from build123d import *
from build123d.topology import SkipClean

# Parameters (mm, degrees)
BOSS_EXTRUDE1_DEPTH     = 1.5875
FILLET1_R               = 6.35
BOSS_EXTRUDE2_DEPTH     = 1.5875
FILLET2_R               = 3.175
CUT_EXTRUDE1_DEPTH      = 107.31034378
CUT_EXTRUDE1_DEPTH_BACK = 107.31034378
SKETCH3_R               = 1.5875


with BuildPart() as part:
    # Sketch1 → Boss-Extrude1 (new, symmetric)
    with SkipClean():  # the faces are left unmerged after this step: merging them gives an invalid solid
        with BuildSketch(Plane(origin=(0, 0, 0), x_dir=(0, 0, -1), z_dir=(1, 0, 0))):
            with BuildLine():
                Line((-38.1, -3.698033758), (-9.463093909, -3.698033758))
                ThreePointArc((-9.463093909, -3.698033758), (-10.16, 0), (-9.463093909, 3.698033758))
                Line((-9.463093909, 3.698033758), (-38.1, 3.698033758))
                ThreePointArc((-38.1, 3.698033758), (-41.798033758, 0), (-38.1, -3.698033758))
            make_face()
            with BuildLine():
                Line((-9.463093909, -3.698033758), (0, -3.698033758))
                ThreePointArc((0, -3.698033758), (-3.698033758, 0), (0, 3.698033758))
                Line((0, 3.698033758), (-9.463093909, 3.698033758))
                ThreePointArc((-9.463093909, 3.698033758), (-10.16, 0), (-9.463093909, -3.698033758))
            make_face()
            with BuildLine():
                Line((-9.463093909, 3.698033758), (0, 3.698033758))
                Line((0, 3.698033758), (9.463093909, 3.698033758))
                ThreePointArc((9.463093909, 3.698033758), (0, 10.16), (-9.463093909, 3.698033758))
            make_face()
            with BuildLine():
                Line((9.463093909, -3.698033758), (0, -3.698033758))
                Line((0, -3.698033758), (-9.463093909, -3.698033758))
                ThreePointArc((-9.463093909, -3.698033758), (0, -10.16), (9.463093909, -3.698033758))
            make_face()
            with BuildLine():
                ThreePointArc((0, 3.698033758), (3.698033758, 0), (0, -3.698033758))
                Line((0, -3.698033758), (9.463093909, -3.698033758))
                ThreePointArc((9.463093909, -3.698033758), (9.984253455, -1.881563962), (10.16, 0))
                ThreePointArc((10.16, 0), (9.984253455, 1.881563962), (9.463093909, 3.698033758))
                Line((9.463093909, 3.698033758), (0, 3.698033758))
            make_face()
            with BuildLine():
                ThreePointArc((10.16, 0), (9.984253455, -1.881563962), (9.463093909, -3.698033758))
                Line((9.463093909, -3.698033758), (101.6, -3.698033758))
                ThreePointArc((101.6, -3.698033758), (105.298033758, 0), (101.6, 3.698033758))
                Line((101.6, 3.698033758), (9.463093909, 3.698033758))
                ThreePointArc((9.463093909, 3.698033758), (9.984253455, 1.881563962), (10.16, 0))
            make_face()
        extrude(amount=BOSS_EXTRUDE1_DEPTH, both=True)

    # Fillet1
    fillet1_edges = [part.edges().sort_by_distance(p)[0] for p in [
        (0, -3.698033758, 9.463093909),
        (0, 3.698033758, 9.463093909),
        (0.79375, 3.698033758, -9.463093909),
        (0.79375, -3.698033758, -9.463093909),
    ]]
    fillet(fillet1_edges, radius=FILLET1_R)

    # Sketch2 → Boss-Extrude2 (add, symmetric)
    with SkipClean():  # the faces are left unmerged after this step: merging them gives an invalid solid
        with BuildSketch(Plane(origin=(0, 0, 0), x_dir=(0, 0, -1), z_dir=(1, 0, 0))):
            with BuildLine():
                Line((105.298033758, 0), (105.298033758, 12.7))
                ThreePointArc((105.298033758, 12.7), (103.756361287, 14.286838394), (102.125679632, 12.79161686))
                Line((102.125679632, 12.79161686), (101.6, 3.698033758))
                ThreePointArc((101.6, 3.698033758), (104.214904747, 2.614904747), (105.298033758, 0))
            make_face()
        extrude(amount=BOSS_EXTRUDE2_DEPTH, both=True)

    # Fillet2
    # the kernel refuses this fillet: 3.175 mm, written as the material it adds along each edge
    with BuildSketch(Plane(origin=(1.5875, 3.698033758, -101.6), x_dir=(0, 0, 1), z_dir=(-1, 0, 0))) as fillet2_piece_1:
        with BuildLine():
            CenterArc((FILLET2_R * 0.943861718873, FILLET2_R), FILLET2_R, 183.308458381, 86.691541619)
            Line((-FILLET2_R * 0.0544715888813, FILLET2_R * 0.942288591865), (0, 0))
            Line((0, 0), (FILLET2_R * 0.943861718873, 0))
        make_face()
    extrude(amount=3.175)

    # Sketch3 → Cut-Extrude1 (cut, two sides: drawn at the far end of the back side and taken through both)
    with BuildSketch(Plane(origin=(1.5875, 0, 0), x_dir=(0, 0, -1), z_dir=(1, 0, 0)).offset(-CUT_EXTRUDE1_DEPTH_BACK)):
        with Locations((-38.1, 0)):
            Circle(SKETCH3_R)
    extrude(amount=CUT_EXTRUDE1_DEPTH + CUT_EXTRUDE1_DEPTH_BACK, mode=Mode.SUBTRACT)


solid = part.part
Check sheet for the modelled part. Datum: model origin and axes. Units: mm. A direction names the side the tool comes from. Coordinates: 2 decimals unless noted, no trailing zeros. Write each loop counter-clockwise with the first axis right and the second up, starting at its lowest first coordinate (ties: lowest second). Pieces come first, ordered by that corner, then holes. Notation, with made-up numbers: M 71,31.5 L 80,31.5 A25 ccw 80,69.5 Z; hole C -24.75,77 d6. An arc over 180 degrees is marked long. Answer as CSV lines item,"result".
Q1. Cross-section at A-A (x = 0.75). Count the separate pieces of the cut face and the enclosed holes in it, then the cut area to 3 significant figures.
Check result:
separate pieces,"1"
enclosed holes,"2"
area,"1,250 mm^2"
Q2. Cross-section at C-C (z = -92.5). Record the boundary of the cut face in (x, y), then the cut area to 3 significant figures.
Check result:
outline,"M -1.59,-3.7 L 1.59,-3.7 L 1.59,3.7 L -1.59,3.7 Z"
area,"23.5 mm^2"
Q3. Material ranges on probe 1 along Y at (x, z) = (0.05, 38.1); probe 2 along Y at (x, z) = (1.3, 22.5); probe 3 along Z at (x, y) = (-1.3, 6), recorded low to high. Write a range as from..to.
Check result:
probe 1,"-3.7..-1.59, 1.59..3.7"
probe 2,"-3.7..3.7"
probe 3,"-105.3..-101.66, -8.21..8.21"
Q4. Set-up check for faces 4 (the face through (0, -3.698, 26)), 5 (the face through (0, -3.698, -57)), 6 (the face through (0, 3.698, 25)), 7 (the face through (0.022, 4.371, -10.255)), 8 (the face through (1.588, 1, -31)): record each of +Z, -Z, +X, -X, +Y, -Y from which the full face is reachable in a straight line by a thin tool's end or side.
Check result:
face 4,"+Z, +X, -X, -Y"
face 5,"-Z, +X, -X, -Y"
face 6,"+Z, +X, -X, +Y"
face 7,"+X, -X, +Y"
face 8,"+Z, -Z, +X, +Y, -Y"
Q5. Mould release check, pull along Z, two halves, no side actions. Record for faces 1 (the face through (0.022, 14.285, -103.791)), 2 (the face through (-0.022, 4.335, 10.328)), 3 (the face through (0.02, 10.16, -0.13)): released by +Z, released by -Z, zero draft, split by the parting line, or undercut.
Check result:
face 1,"split by the parting line"
face 2,"released by +Z"
face 3,"undercut"
Q6. Cross-section at B-B (y = 8). Record the boundary of the cut face in (x, z), then the cut area to 3 significant figures.
Check result:
outline,"M -1.59,-105.3 L 1.59,-105.3 L 1.59,-101.85 L -1.59,-101.85 Z; M -1.59,-6.26 L 1.59,-6.26 L 1.59,6.26 L -1.59,6.26 Z"
area,"50.7 mm^2"
Q7. Go/stop test with flat-tipped pins: pin 1 (1 mm diameter, centred on x = 1, z = 12.5, fed in from -Y); pin 2 (1 mm diameter, centred on x = 0, z = -35, fed in from +Y); pin 3 (1.6 mm diameter, centred on x = 0, z = 20.5, fed in from -Y); pin 4 (2 mm diameter, centred on y = 6.5, z = -64.5, fed in from +X). Record where each tip stops, or that it passes through.
Check result:
pin 1,"y = -3.79"
pin 2,"y = 3.7"
pin 3,"y = -3.7"
pin 4,"through"
